Geometry check sheet. Reference: the model listing, model coordinates, mm. Round coordinates to 2 decimals unless told otherwise and drop trailing zeros. Loops run counter-clockwise (first coordinate to the right, second up) from the corner with the lowest first, then second, coordinate; pieces in that order, holes last. Notation, with made-up numbers: (6.5, 43.5) -> (38.5, 43.5) arc R17 ccw to (38.5, 69.5) -> close; hole circle Ø3 at (56.5, -1). An arc over 180 degrees is marked (long way). Use a Markdown table: item, result. Add a question column.
Q1. Sectioned sample at C-C, the plane y = -1.75. Enter the section's corners in (x, z), then the cut area to 3 significant figures.
Q2. Sectioned sample at B-B, the plane x = 0. Enter the section's corners in (y, z).
Q3. Sectioned sample at A-A, the plane z = 3. Enter the section's corners in (x, y), then the cut area to 3 significant figures.
Q4. Material ranges on L1, parallel to Z at x = 0, y = -5; L2, parallel to X at y = -1, z = -0.5; L3, parallel to Z at x = -1, y = -2.5, recorded low to high.
```python
from build123d import *

# Parameters (mm, degrees)
F0_R     = 5.5
F1_DEPTH = 8


with BuildPart() as f1:
    # F0 (on Front) → F1 (new body)
    with BuildSketch(Plane.XZ):
        with BuildLine():
            Line((-15, -15), (15, -15))
            Line((15, -15), (15, 13))
            ThreePointArc((15, 13), (14.414214, 14.414214), (13, 15))
            Line((13, 15), (-13, 15))
            ThreePointArc((-13, 15), (-14.414214, 14.414214), (-15, 13))
            Line((-15, 13), (-15, -15))
        make_face()
        with Locations((0, 3)):
            Circle(F0_R, mode=Mode.SUBTRACT)
    extrude(amount=F1_DEPTH)


solid = f1.part
```
Values:
| question | item | result |
|---|---|---|
| 1 | outline | (-15, -15) -> (15, -15) -> (15, 13) arc R2 ccw to (13, 15) -> (-13, 15) arc R2 ccw to (-15, 13) -> close; hole circle Ø11 at (0, 3) |
| 1 | area | 803 mm^2 |
| 2 | outline | (-8, -15) -> (0, -15) -> (0, -2.5) -> (-8, -2.5) -> close; (-8, 8.5) -> (0, 8.5) -> (0, 15) -> (-8, 15) -> close |
| 3 | outline | (-15, -8) -> (-5.5, -8) -> (-5.5, 0) -> (-15, 0) -> close; (5.5, -8) -> (15, -8) -> (15, 0) -> (5.5, 0) -> close |
| 3 | area | 152 mm^2 |
| 4 | L1 | -15 to -2.5, 8.5 to 15 |
| 4 | L2 | -15 to -4.24, 4.24 to 15 |
| 4 | L3 | -15 to -2.41, 8.41 to 15 |
